Part model, mm, in its own coordinate system. Face numbers are marked on the shaded views. A direction names the side the tool comes from. Round coordinates to 2 decimals unless told otherwise and drop trailing zeros. Loops run counter-clockwise (first coordinate to the right, second up) from the corner with the lowest first, then second, coordinate; pieces in that order, holes last.
Autodesk Inventor part; units mm, degrees
ref_plane "YZ Plane" through (0, 0, 0) normal (1, 0, 0) x (0, 1, 0)
ref_plane "XZ Plane" through (0, 0, 0) normal (0, 1, 0) x (-1, 0, 0)
ref_plane "XY Plane" through (0, 0, 0) normal (0, 0, 1) x (1, 0, 0)
sketch "Sketch1" plane through (0, 0, 0) normal (0, 1, 0) x (-1, 0, 0)
  circle A0 centre (0, 0) radius 2
  circle A1 centre (0, 0) radius 5.9473
  line L0 (5.3451, 5.9473) -> (2.9816, 5.146)
  line L1 (5.3451, 5.9473) -> (4.9023, 3.3673)
  line L2 (1.6553, 7.8231) -> (0.0091, 5.9473)
  line L3 (1.6553, 7.8231) -> (2.5618, 5.3673)
  line L4 (-2.478, 7.6027) -> (-2.9658, 5.1551)
  line L5 (-2.478, 7.6027) -> (-0.465, 5.9291)
  line L6 (-5.9473, 5.3451) -> (-5.146, 2.9816)
  line L7 (-5.9473, 5.3451) -> (-3.3673, 4.9023)
  line L8 (-7.8231, 1.6553) -> (-5.9473, 0.0091)
  line L9 (-7.8231, 1.6553) -> (-5.3673, 2.5618)
  line L10 (-7.6027, -2.478) -> (-5.1551, -2.9658)
  line L11 (-7.6027, -2.478) -> (-5.9291, -0.465)
  line L12 (-5.3451, -5.9473) -> (-2.9816, -5.146)
  line L13 (-5.3451, -5.9473) -> (-4.9023, -3.3673)
  line L14 (-1.6553, -7.8231) -> (-0.0091, -5.9473)
  line L15 (-1.6553, -7.8231) -> (-2.5618, -5.3673)
  line L16 (2.478, -7.6027) -> (2.9658, -5.1551)
  line L17 (2.478, -7.6027) -> (0.465, -5.9291)
  line L18 (5.9473, -5.3451) -> (5.146, -2.9816)
  line L19 (5.9473, -5.3451) -> (3.3673, -4.9023)
  line L20 (7.8231, -1.6553) -> (5.9473, -0.0091)
  line L21 (7.8231, -1.6553) -> (5.3673, -2.5618)
  line L22 (7.6027, 2.478) -> (5.1551, 2.9658)
  line L23 (7.6027, 2.478) -> (5.9291, 0.465)
  dimension "d0" = 4
  dimension "d3" = 360
extrude "Extrusion1" add sketch "Sketch1" along normal blind 3
properties part number "gir"
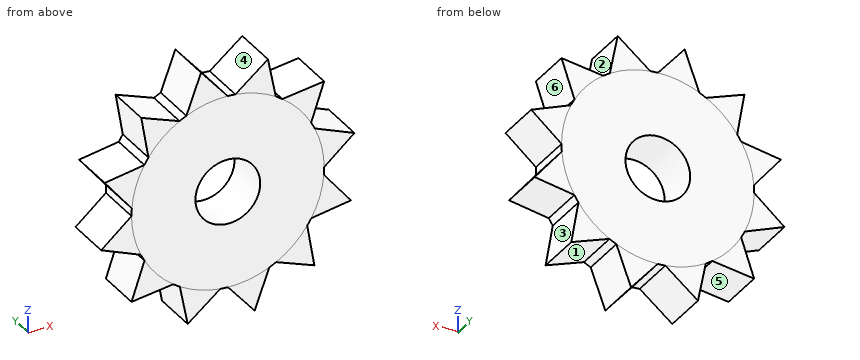
1) Mould opens along Z. For the marked faces 1, 2 and 3 say: released by +Z, released by -Z, zero draft, split by the parting line, or undercut.
Values:
face 1: released by -Z
face 2: released by +Z
face 3: undercut
2) Tool access for the marked faces 4, 5 and 6: list every direction of +Z, -Z, +X, -X, +Y, -Y with a clear straight run to the whole face (end or side of a thin tool).
Values:
face 4: +Z, +Y, -Y
face 5: -Z, +Y, -Y
face 6: +X, +Y, -Y
3) Drop flat-ended pins along their axis: pin 1 Ø1.5 at (y, z) = (2, 0.5) entering from +X; pin 2 Ø1.5 at (x, y) = (2, 1.5) entering from +Z; pin 3 Ø8 at (x, z) = (-4, 1) entering from -Y. Give the stop position or say it passes through.
Values:
pin 1: stops at x = 7.36
pin 2: stops at z = 7.6
pin 3: stops at y = 0
4) Slice it at A-A, the plane x = 6.5. Give the cut face in (y, z).
Values:
outline: (0, -2.7) - (3, -2.7) - (3, -1.15) - (0, -1.15) - close; (0, 0.49) - (3, 0.49) - (3, 2.14) - (0, 2.14) - close
5) Slice it at C-C, the plane z = 4.5. Give the cut face in (x, y).
Values:
outline: (-5.1, 0) - (5.66, 0) - (5.66, 3) - (-5.1, 3) - close
6) Slice it at B-B, the plane x = -1.25. Give the cut face in (y, z).
Values:
outline: (0, -6.58) - (3, -6.58) - (3, -1.56) - (0, -1.56) - close; (0, 1.56) - (3, 1.56) - (3, 7.36) - (0, 7.36) - close
7) Wall check: line 1 along Z through (x, y) = (-6.5, 0.75); line 2 along Z through (x, y) = (-1.5, 2.2). Give the ranges that are in metal, low to high.
Values:
line 1: z = -2.14 to -0.49, 1.15 to 2.7
line 2: z = -6.79 to -1.32, 1.32 to 7.65
